Check sheet for the modelled part. Datum: model origin and axes. Units: mm. A direction names the side the tool comes from. Coordinates: 2 decimals unless noted, no trailing zeros. Write each loop counter-clockwise with the first axis right and the second up, starting at its lowest first coordinate (ties: lowest second). Pieces come first, ordered by that corner, then holes. Notation, with made-up numbers: (63, 69) -> (71, 69) arc R23 cw to (71, 98) -> close; hole circle Ø10 at (-39, 6.25). An arc over 180 degrees is marked (long way). Put each result on its own line as item: value.
```python
from build123d import *

# Parameters (mm, degrees)
SKETCH1_R           = 1.7
BOSS_EXTRUDE1_DEPTH = 6
FILLET1_R           = 10
SKETCH1_4_R         = 1.7
BOSS_EXTRUDE2_DEPTH = 10


with BuildPart() as part:
    # Sketch1 → Boss-Extrude1 (new body)
    with BuildSketch(Plane(origin=(0, 0, 0), x_dir=(1, 0, 0), z_dir=(0, 1, 0))):
        with BuildLine():
            Line((-72.831998462, 89.802561211), (-13.029437252, 30))
            Line((-13.029437252, 30), (13.029437252, 30))
            Line((13.029437252, 30), (72.831998462, 89.802561211))
            ThreePointArc((72.831998462, 89.802561211), (89.802561211, 89.802561211), (89.802561211, 72.831998462))
            Line((89.802561211, 72.831998462), (30, 13.029437252))
            Line((30, 13.029437252), (30, -13.029437252))
            Line((30, -13.029437252), (89.802561211, -72.831998462))
            ThreePointArc((89.802561211, -72.831998462), (89.802561211, -89.802561211), (72.831998462, -89.802561211))
            Line((72.831998462, -89.802561211), (13.029437252, -30))
            Line((13.029437252, -30), (-13.029437252, -30))
            Line((-13.029437252, -30), (-72.831998462, -89.802561211))
            ThreePointArc((-72.831998462, -89.802561211), (-89.802561211, -89.802561211), (-89.802561211, -72.831998462))
            Line((-89.802561211, -72.831998462), (-30, -13.029437252))
            Line((-30, -13.029437252), (-30, 13.029437252))
            Line((-30, 13.029437252), (-89.802561211, 72.831998462))
            ThreePointArc((-89.802561211, 72.831998462), (-89.802561211, 89.802561211), (-72.831998462, 89.802561211))
        make_face()
        with Locations(Location((67.787488849, 67.787488849, 0), (0, 0, 270))):
            Circle(SKETCH1_R, mode=Mode.SUBTRACT)
        with Locations(Location((58.807232728, 58.807232728, 0), (0, 0, 270))):
            Circle(SKETCH1_R, mode=Mode.SUBTRACT)
        with Locations(Location((49.826976607, 49.826976607, 0), (0, 0, 270))):
            Circle(SKETCH1_R, mode=Mode.SUBTRACT)
        with Locations(Location((40.846720486, 40.846720486, 0), (0, 0, 270))):
            Circle(SKETCH1_R, mode=Mode.SUBTRACT)
        with Locations(Location((31.866464365, 31.866464365, 0), (0, 0, 270))):
            Circle(SKETCH1_R, mode=Mode.SUBTRACT)
        with Locations(Location((67.787488849, -67.787488849, 0), (0, 0, 90))):
            Circle(SKETCH1_R, mode=Mode.SUBTRACT)
        with Locations(Location((58.807232728, -58.807232728, 0), (0, 0, 90))):
            Circle(SKETCH1_R, mode=Mode.SUBTRACT)
        with Locations(Location((49.826976607, -49.826976607, 0), (0, 0, 90))):
            Circle(SKETCH1_R, mode=Mode.SUBTRACT)
        with Locations(Location((40.846720486, -40.846720486, 0), (0, 0, 90))):
            Circle(SKETCH1_R, mode=Mode.SUBTRACT)
        with Locations(Location((31.866464365, -31.866464365, 0), (0, 0, 90))):
            Circle(SKETCH1_R, mode=Mode.SUBTRACT)
        with Locations(Location((-67.787488849, 67.787488849, 0), (0, 0, 90))):
            Circle(SKETCH1_R, mode=Mode.SUBTRACT)
        with Locations(Location((-58.807232728, 58.807232728, 0), (0, 0, 90))):
            Circle(SKETCH1_R, mode=Mode.SUBTRACT)
        with Locations(Location((-31.866464365, 31.866464365, 0), (0, 0, 90))):
            Circle(SKETCH1_R, mode=Mode.SUBTRACT)
        with Locations(Location((-49.826976607, 49.826976607, 0), (0, 0, 90))):
            Circle(SKETCH1_R, mode=Mode.SUBTRACT)
        with Locations(Location((-40.846720486, 40.846720486, 0), (0, 0, 90))):
            Circle(SKETCH1_R, mode=Mode.SUBTRACT)
        with Locations(Location((-31.866464365, -31.866464365, 0), (0, 0, 270))):
            Circle(SKETCH1_R, mode=Mode.SUBTRACT)
        with Locations(Location((-58.807232728, -58.807232728, 0), (0, 0, 270))):
            Circle(SKETCH1_R, mode=Mode.SUBTRACT)
        with Locations(Location((-40.846720486, -40.846720486, 0), (0, 0, 270))):
            Circle(SKETCH1_R, mode=Mode.SUBTRACT)
        with Locations(Location((-49.826976607, -49.826976607, 0), (0, 0, 270))):
            Circle(SKETCH1_R, mode=Mode.SUBTRACT)
        with Locations(Location((-67.787488849, -67.787488849, 0), (0, 0, 270))):
            Circle(SKETCH1_R, mode=Mode.SUBTRACT)
    extrude(amount=BOSS_EXTRUDE1_DEPTH)

    # Fillet1
    fillet1_edges = [part.edges().sort_by_distance(p)[0] for p in [
        (-13.029437252, 3, -30),
        (13.029437252, 3, -30),
        (30, 3, -13.029437252),
        (30, 3, 13.029437252),
        (13.029437252, 3, 30),
        (-13.029437252, 3, 30),
        (-30, 3, 13.029437252),
        (-30, 3, -13.029437252),
    ]]
    fillet(fillet1_edges, radius=FILLET1_R)

    # Sketch1_4 → Boss-Extrude2 (add)
    with BuildSketch(Plane(origin=(0, 0, 0), x_dir=(1, 0, 0), z_dir=(0, 1, 0))):
        with BuildLine():
            Line((-72.831998462, 89.802561211), (-13.029437252, 30))
            Line((-13.029437252, 30), (13.029437252, 30))
            Line((13.029437252, 30), (72.831998462, 89.802561211))
            ThreePointArc((72.831998462, 89.802561211), (89.802561211, 89.802561211), (89.802561211, 72.831998462))
            Line((89.802561211, 72.831998462), (30, 13.029437252))
            Line((30, 13.029437252), (30, -13.029437252))
            Line((30, -13.029437252), (89.802561211, -72.831998462))
            ThreePointArc((89.802561211, -72.831998462), (89.802561211, -89.802561211), (72.831998462, -89.802561211))
            Line((72.831998462, -89.802561211), (13.029437252, -30))
            Line((13.029437252, -30), (-13.029437252, -30))
            Line((-13.029437252, -30), (-72.831998462, -89.802561211))
            ThreePointArc((-72.831998462, -89.802561211), (-89.802561211, -89.802561211), (-89.802561211, -72.831998462))
            Line((-89.802561211, -72.831998462), (-30, -13.029437252))
            Line((-30, -13.029437252), (-30, 13.029437252))
            Line((-30, 13.029437252), (-89.802561211, 72.831998462))
            ThreePointArc((-89.802561211, 72.831998462), (-89.802561211, 89.802561211), (-72.831998462, 89.802561211))
        make_face()
        with Locations(Location((67.787488849, 67.787488849, 0), (0, 0, 270))):
            Circle(SKETCH1_4_R, mode=Mode.SUBTRACT)
        with Locations(Location((58.807232728, 58.807232728, 0), (0, 0, 270))):
            Circle(SKETCH1_4_R, mode=Mode.SUBTRACT)
        with Locations(Location((49.826976607, 49.826976607, 0), (0, 0, 270))):
            Circle(SKETCH1_4_R, mode=Mode.SUBTRACT)
        with Locations(Location((40.846720486, 40.846720486, 0), (0, 0, 270))):
            Circle(SKETCH1_4_R, mode=Mode.SUBTRACT)
        with Locations(Location((31.866464365, 31.866464365, 0), (0, 0, 270))):
            Circle(SKETCH1_4_R, mode=Mode.SUBTRACT)
        with Locations(Location((67.787488849, -67.787488849, 0), (0, 0, 90))):
            Circle(SKETCH1_4_R, mode=Mode.SUBTRACT)
        with Locations(Location((58.807232728, -58.807232728, 0), (0, 0, 90))):
            Circle(SKETCH1_4_R, mode=Mode.SUBTRACT)
        with Locations(Location((49.826976607, -49.826976607, 0), (0, 0, 90))):
            Circle(SKETCH1_4_R, mode=Mode.SUBTRACT)
        with Locations(Location((40.846720486, -40.846720486, 0), (0, 0, 90))):
            Circle(SKETCH1_4_R, mode=Mode.SUBTRACT)
        with Locations(Location((31.866464365, -31.866464365, 0), (0, 0, 90))):
            Circle(SKETCH1_4_R, mode=Mode.SUBTRACT)
        with Locations(Location((-67.787488849, 67.787488849, 0), (0, 0, 90))):
            Circle(SKETCH1_4_R, mode=Mode.SUBTRACT)
        with Locations(Location((-58.807232728, 58.807232728, 0), (0, 0, 90))):
            Circle(SKETCH1_4_R, mode=Mode.SUBTRACT)
        with Locations(Location((-31.866464365, 31.866464365, 0), (0, 0, 90))):
            Circle(SKETCH1_4_R, mode=Mode.SUBTRACT)
        with Locations(Location((-49.826976607, 49.826976607, 0), (0, 0, 90))):
            Circle(SKETCH1_4_R, mode=Mode.SUBTRACT)
        with Locations(Location((-40.846720486, 40.846720486, 0), (0, 0, 90))):
            Circle(SKETCH1_4_R, mode=Mode.SUBTRACT)
        with Locations(Location((-31.866464365, -31.866464365, 0), (0, 0, 270))):
            Circle(SKETCH1_4_R, mode=Mode.SUBTRACT)
        with Locations(Location((-58.807232728, -58.807232728, 0), (0, 0, 270))):
            Circle(SKETCH1_4_R, mode=Mode.SUBTRACT)
        with Locations(Location((-40.846720486, -40.846720486, 0), (0, 0, 270))):
            Circle(SKETCH1_4_R, mode=Mode.SUBTRACT)
        with Locations(Location((-49.826976607, -49.826976607, 0), (0, 0, 270))):
            Circle(SKETCH1_4_R, mode=Mode.SUBTRACT)
        with Locations(Location((-67.787488849, -67.787488849, 0), (0, 0, 270))):
            Circle(SKETCH1_4_R, mode=Mode.SUBTRACT)
    extrude(amount=BOSS_EXTRUDE2_DEPTH)


solid = part.part
```
Q1. Cross-section at D-D (x = 24). Record the cut outline in (y, z).
Recorded:
outline: (0, -40.97) -> (10, -40.97) -> (10, 40.97) -> (0, 40.97) -> close
Q2. Cross-section at B-B (x = 75.5). Record the cut outline in (y, z).
Recorded:
outline: (0, -91.81) -> (10, -91.81) -> (10, -58.53) -> (0, -58.53) -> close; (0, 58.53) -> (10, 58.53) -> (10, 91.81) -> (0, 91.81) -> close
Q3. Material ranges on line 1 along Z through (x, y) = (31.5, 4); line 2 along Z through (x, y) = (-30.5, 9); line 3 along X through (y, z) = (1.75, 58.5), recorded low to high.
Recorded:
line 1: z = -48.47 to -33.53, -30.21 to -14.16, 14.16 to 30.21, 33.53 to 48.47
line 2: z = -47.47 to -32.88, -30.86 to -13.53, 13.53 to 30.86, 32.88 to 47.47
line 3: x = -75.47 to -60.48, -57.14 to -41.53, 41.53 to 57.14, 60.48 to 75.47
Q4. Depth check by flat-ended pin: P1, Ø2, axis at y = 8, z = 4, coming from the -X side; P2, Ø5, axis at y = 3.5, z = -6.5, coming from the +X side; P3, Ø3, axis at x = -4.5, y = 7.5, coming from the +Z side. Enter the tip coordinate at first touch or a pass-through.
Recorded:
P1: stops at x = -30
P2: stops at x = 30
P3: stops at z = 30
Q5. Tool access check on faces 4 (the cylindrical face through (89.6, 4.9, -90)), 5 (the cylindrical face through (-12.76, 3.04, -30.78)), 6 (the cylindrical face through (30.78, 3.04, -12.76)), 7 (the cylindrical face through (12.66, 3.04, 30.74)), 8 (the cylindrical face through (-30.74, 3.04, 12.66)). Record the directions out of +Z, -Z, +X, -X, +Y, -Y that give a thin tool (end or side, any length) a straight path to the whole face; none if there is none.
Recorded:
face 4: +Y, -Y
face 5: -Z, +Y, -Y
face 6: +X, +Y, -Y
face 7: +Z, +Y, -Y
face 8: -X, +Y, -Y
Q6. Mould release check, pull along X, two halves, no side actions. Record for faces 1 (the flat face through (-60.32, 4.93, 43.35)), 2 (the flat face through (59.48, 4.93, 42.51)), 3 (the cylindrical face through (12.66, 3.04, -30.74)): released by +X, released by -X, zero draft, split by the parting line, or undercut.
Recorded:
face 1: released by -X
face 2: released by +X
face 3: undercut
Q7. Cross-section at C-C (y = 3.5). State how many separate pieces and enclosed holes the cut face has, plus the area to 3 significant figures.
Recorded:
separate pieces: 1
enclosed holes: 20
area: 11,900 mm2
Q8. Cross-section at A-A (z = -79.5). Record the cut outline in (x, y), plus the area to 3 significant figures.
Recorded:
outline: (-93.18, 0) -> (-62.53, 0) -> (-62.53, 10) -> (-93.18, 10) -> close; (62.53, 0) -> (93.18, 0) -> (93.18, 10) -> (62.53, 10) -> close
area: 613 mm2
